from build123d import *

# Parameters (mm, degrees)
F0_R     = 10.16
F1_DEPTH = 3.175
F2_R     = 7.62
F3_DEPTH = 6.35
F4_R     = 2.54
F5_DEPTH = 9.525


with BuildPart() as f1:
    # F0 (on Top) → F1 (new body)
    with BuildSketch(Plane.XY):
        Circle(F0_R)
    extrude(amount=F1_DEPTH)

    # F2 (on face) → F3 (join)
    with BuildSketch(Plane.XY.offset(3.175)):
        Circle(F2_R)
    extrude(amount=F3_DEPTH)

    # F4 (on face) → F5 (cut, through all)
    with BuildSketch(Plane.XY.offset(9.525)):
        Circle(F4_R)
    extrude(amount=-F5_DEPTH, mode=Mode.SUBTRACT)


solid = f1.part
Work out the finished part from the listing and answer in its coordinate system (mm). A direction names the side the tool comes from. Round coordinates to 2 decimals unless told otherwise and drop trailing zeros. Write each loop counter-clockwise with the first axis right and the second up, starting at its lowest first coordinate (ties: lowest second). Pieces come first, ordered by that corner, then holes. Notation, with made-up numbers: (-8.75, 6.5) -> (18.25, 6.5) arc R9 cw to (18.25, 23.5) -> close; hole circle Ø11 at (79, 28.5). An arc over 180 degrees is marked (long way). Answer as CSV lines item,"result". Start each with the question number.
(1) Each of these flat-tipped pins is pushed along its axis until it touches: pin 1 (8 mm diameter, centred on x = -0.5, y = 1, fed in from +Z) (3 decimals); pin 2 (1 mm diameter, centred on y = -5.5, z = 6, fed in from -X); pin 3 (4 mm diameter, centred on y = -3, z = 7, fed in from -X); pin 4 (1.5 mm diameter, centred on x = -4, y = 7.5, fed in from +Z) (3 decimals). Where does it stop, or does it pass through?
(2) The part is cut by section C-C, the plane z = 4. Give the vertices of the cut face in (x, y).
(3) The part is cut by section A-A, the plane x = 0. Give the vertices of the cut face in (y, z) (3 decimals), then the cut area to 3 significant figures.
(4) A tool of negligible diameter and unlimited length cuts with its end or side. For faces 1 (the flat face through (-2, 2, 9.525)), 2 (the cylindrical face through (-1.65, -7.44, 6.31)), from which of +Z, -Z, +X, -X, +Y, -Y can it reach the whole face along a straight path? Write none if from no direction.
(5) The part is cut by section D-D, the plane y = -4.75. Give the vertices of the cut face in (x, z) (3 decimals).
(6) The mould has two halves that part along X. Classify faces 3 (the cylindrical face through (-0.33, 2.52, 4.83)), 4 (the flat face through (1, 8, 3.175)), 5 (the cylindrical face through (-1.323, 10.074, 1.565)): +X half, -X half, draft (parallel to the pull), parting line (faces both ways), or undercut.
(7) Find the intervals of material crossed by probe 1 along Y at (x, z) = (0, 5); probe 2 along X at (y, z) = (1.5, 2.25); probe 3 along Z at (x, y) = (6.5, -6) (3 decimals), in increasing order.
Output values:
1,pin 1,"stops at z = 9.525"
1,pin 2,"stops at x = -5.75"
1,pin 3,"stops at x = -7.55"
1,pin 4,"stops at z = 3.175"
2,outline,"circle Ø15.24 at (0, 0); hole circle Ø5.08 at (0, 0)"
3,outline,"(-10.16, 0) -> (-2.54, 0) -> (-2.54, 9.525) -> (-7.62, 9.525) -> (-7.62, 3.175) -> (-10.16, 3.175) -> close; (2.54, 0) -> (10.16, 0) -> (10.16, 3.175) -> (7.62, 3.175) -> (7.62, 9.525) -> (2.54, 9.525) -> close"
3,area,"113 mm²"
4,face 1,"+Z, +X, -X, +Y, -Y"
4,face 2,"+Z"
5,outline,"(-8.981, 0) -> (8.981, 0) -> (8.981, 3.175) -> (5.958, 3.175) -> (5.958, 9.525) -> (-5.958, 9.525) -> (-5.958, 3.175) -> (-8.981, 3.175) -> close"
6,face 3,"undercut"
6,face 4,"draft"
6,face 5,"parting line"
7,probe 1,"y = -7.62 to -2.54, 2.54 to 7.62"
7,probe 2,"x = -10.05 to -2.05, 2.05 to 10.05"
7,probe 3,"z = 0 to 3.175"
